```python
from build123d import *

# Parameters (mm, degrees)
EXTRUDE_2_OUTLINE_W   = 140.770566096
EXTRUDE_2_OUTLINE_H   = 72
EXTRUDE_2_OUTLINE_R   = 1.7
EXTRUDE_2_OUTLINE_W_2 = 4.7
EXTRUDE_2_OUTLINE_H_2 = 21.788461539
EXTRUDE_2_OUTLINE_R_2 = 2.2
EXTRUDE_2_DEPTH       = 7
SKETCH_2_R            = 2.9
SKETCH_2_R_2          = 4.8
CUT_EXTRUDE_1_DEPTH   = 3
EXTRUDE_3_DEPTH       = 5
FILLET_1_R            = 3
SKETCH_4_R            = 2
CUT_EXTRUDE_2_DEPTH   = 159.482615774


# Read off the part's stored shape, not the designer's step: 填料-伸長2
with BuildPart() as part:
    # 填料-伸長2 outline → 填料-伸長2 (new body)
    with BuildSketch(Plane.XZ.offset(5.158117597)):
        with Locations((-64.32262294, -19.915289206)):
            Rectangle(EXTRUDE_2_OUTLINE_W, EXTRUDE_2_OUTLINE_H)
        with Locations((-129.707905988, -45.915289206)):
            Circle(EXTRUDE_2_OUTLINE_R, mode=Mode.SUBTRACT)
        with Locations((-83.937339892, -45.915289206)):
            Circle(EXTRUDE_2_OUTLINE_R, mode=Mode.SUBTRACT)
        with Locations((-40.175495169, -19.915289206)):
            Rectangle(EXTRUDE_2_OUTLINE_W_2, EXTRUDE_2_OUTLINE_H_2, mode=Mode.SUBTRACT)
        with Locations((-129.707905988, 6.084710794)):
            Circle(EXTRUDE_2_OUTLINE_R, mode=Mode.SUBTRACT)
        with Locations((-83.937339892, 6.084710794)):
            Circle(EXTRUDE_2_OUTLINE_R, mode=Mode.SUBTRACT)
        with Locations((-6.29428449, -19.915289206)):
            Circle(EXTRUDE_2_OUTLINE_R_2, mode=Mode.SUBTRACT)
    extrude(amount=EXTRUDE_2_DEPTH)

    # 草圖2 → 除料-伸長1 (cut)
    with BuildSketch(Plane.XZ.offset(12.158117597)):
        with Locations(Location((-129.707905988, -45.915289206, 0), (0, 0, 270))):
            Circle(SKETCH_2_R)
        with Locations(Location((-129.707905988, 6.084710794, 0), (0, 0, 270))):
            Circle(SKETCH_2_R)
        with Locations(Location((-83.937339892, 6.084710794, 0), (0, 0, 270))):
            Circle(SKETCH_2_R)
        with Locations(Location((-83.937339892, -45.915289206, 0), (0, 0, 270))):
            Circle(SKETCH_2_R)
        with Locations(Location((-6.29428449, -19.915289206, 0), (0, 0, 270))):
            Circle(SKETCH_2_R_2)
    extrude(amount=-CUT_EXTRUDE_1_DEPTH, mode=Mode.SUBTRACT)

    # 草圖3 → 填料-伸長3 (add)
    with BuildSketch(Plane.ZY.offset(134.707905988)):
        Polygon((0.484710794, -5.158117597), (-40.315289206, -5.158117597), (-40.315289206, 0.441882403), (-40.915289206, 0.441882403), (-50.315289206, 0.441882403), (-50.315289206, 49.841882403), (10.484710794, 49.841882403), (10.484710794, 0.441882403), (1.084710794, 0.441882403), (0.484710794, 0.441882403), align=None)
    extrude(amount=-EXTRUDE_3_DEPTH)

    # 圓角1
    fillet_1_edges = [part.edges().sort_by_distance(p)[0] for p in [
        (-129.707905988, -5.158117597, -19.915289206),
    ]]
    fillet(fillet_1_edges, radius=FILLET_1_R)

    # 草圖4 → 除料-伸長2 (cut, through all)
    with BuildSketch(Plane.XZ.offset(12.158117597)):
        with Locations(Location((-58.937339892, 6.084710794, 0), (0, 0, 270))):
            Circle(SKETCH_4_R)
        with Locations(Location((-13.937339892, 6.084710794, 0), (0, 0, 270))):
            Circle(SKETCH_4_R)
        with Locations(Location((-13.937339892, -45.915289206, 0), (0, 0, 270))):
            Circle(SKETCH_4_R)
        with Locations(Location((-58.937339892, -45.915289206, 0), (0, 0, 270))):
            Circle(SKETCH_4_R)
    extrude(amount=-CUT_EXTRUDE_2_DEPTH, mode=Mode.SUBTRACT)


solid = part.part
```
The model under review builds one solid part; all positions refer to its coordinate system, in mm. A direction names the side the tool comes from. Give positions to 0.01 mm unless a question says otherwise; leave off trailing zeros. Write each loop counter-clockwise with the first axis right and the second up, starting at its lowest first coordinate (ties: lowest second). Pieces come first, ordered by that corner, then holes. Notation, with made-up numbers: M -38,32.25 L 20,32.25 A31 cw 20,70.25 Z; hole C -3.5,-25 d4. An arc over 180 degrees is marked long. Answer in a Markdown table with one row per item.
Item 1: Add section B-B on y = 25.5. Give the boundary of the cut face in (x, z).
Check sheet entries:
| item | result |
|---|---|
| outline | M -134.71,-50.32 L -129.71,-50.32 L -129.71,10.48 L -134.71,10.48 Z |
Item 2: Add section A-A on z = -37. Give the boundary of the cut face in (x, y).
Check sheet entries:
| item | result |
|---|---|
| outline | M -134.71,-12.16 L 6.06,-12.16 L 6.06,-5.16 L -126.71,-5.16 A3 cw -129.71,-2.16 L -129.71,49.84 L -134.71,49.84 Z |
Item 3: For P1, Ø6.5, axis at x = -83.5, z = -46.5, coming from the -Y side; P2, Ø2.5, axis at x = -13.94, z = 6.08, coming from the +Y side; P3, Ø8.5, axis at x = -6.29, z = -19.92, coming from the +Y side; P4, Ø4.5, axis at x = -132.5, y = -2.5, coming from the +Z side, all flat-tipped, find the tip position at first contact; note any pin that passes through.
Check sheet entries:
| item | result |
|---|---|
| P1 | y = -12.16 |
| P2 | through |
| P3 | y = -5.16 |
| P4 | z = 0.48 |
Item 4: Add section C-C on x = -91. Give the boundary of the cut face in (y, z).
Check sheet entries:
| item | result |
|---|---|
| outline | M -12.16,-55.92 L -5.16,-55.92 L -5.16,16.08 L -12.16,16.08 Z |
Item 5: For line 1 along X through (y, z) = (24, -13); line 2 along Y through (x, z) = (-81.5, -3.5); line 3 along X through (y, z) = (-4.5, -29), list the stretches that pass through material, from the lowest coordinate up.
Check sheet entries:
| item | result |
|---|---|
| line 1 | -134.71 to -129.71 |
| line 2 | -12.16 to -5.16 |
| line 3 | -134.71 to -128.58 |
Item 6: Draft analysis for pull direction Y (two halves, no side actions). For faces 1 (the face through (-132, 0.442, -45)), 2 (the face through (-65, -9, 16.085)), 3 (the face through (-132, -9.158, -46)), 4 (the face through (-132, 49.842, -20)), state which applies: +Y half, -Y half, draft (parallel to the pull), parting line (faces both ways), or undercut.
Check sheet entries:
| item | result |
|---|---|
| face 1 | undercut |
| face 2 | draft |
| face 3 | -Y half |
| face 4 | +Y half |
Item 7: Tool access review of faces 5 (the face through (-132, 0.442, 5)), 6 (the face through (-132, -2, -40.315)), 7 (the face through (-40, -9, -30.81)), 8 (the face through (-81.06, -10.68, 6.46)), 9 (the face through (-134.708, 19, -20)): name each direction out of +Z, -Z, +X, -X, +Y, -Y from which nothing blocks a thin tool from reaching the whole face with its end or side.
Check sheet entries:
| item | result |
|---|---|
| face 5 | +Z, +X, -X |
| face 6 | -Z, +X, -X |
| face 7 | +Y, -Y |
| face 8 | -Y |
| face 9 | +Z, -Z, -X, +Y, -Y |
